Here's how the part is built. I have some questions about the finished solid (model axes, mm). Face numbers are marked on the shaded views. A direction names the side the tool comes from. Round coordinates to 2 decimals unless told otherwise and drop trailing zeros. Write each loop counter-clockwise with the first axis right and the second up, starting at its lowest first coordinate (ties: lowest second). Pieces come first, ordered by that corner, then holes. Notation, with made-up numbers: (85.25, -7.5) -> (127.25, -7.5) arc R14 ccw to (127.25, 19.5) -> close; hole circle Ø11 at (14.5, -2). An arc over 180 degrees is marked (long way). Answer in a Markdown table with one row per item.
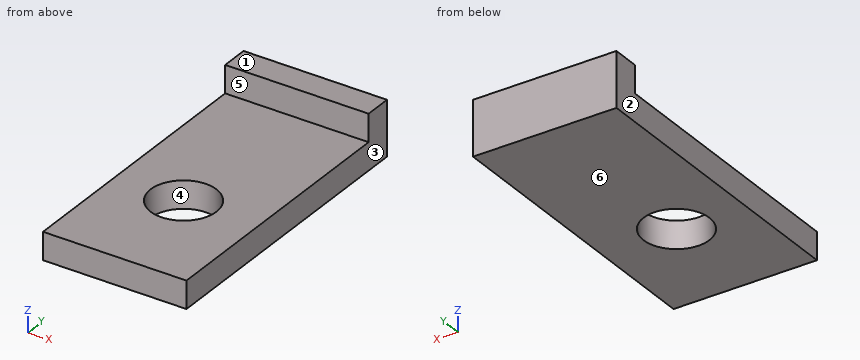
Autodesk Fusion 360 part; units mm, degrees
sketch "Esboço1" plane through (0, 0, 0) normal (0, 0, 1) x (1, 0, 0)
  line L0 (9, 9.5) -> (-9, 9.5)
  line L1 (-9, 9.5) -> (-9, -9.5)
  line L2 (-9, -9.5) -> (9, -9.5)
  line L3 (9, -9.5) -> (9, 9.5)
  line L4 (9, 9.5) -> (-9, -9.5) construction
  line L5 (-9, 9.5) -> (9, -9.5) construction
  line L6 (-7, -7.5) -> (7, -7.5)
  line L7 (7, -7.5) -> (7, 7.5)
  line L8 (7, 7.5) -> (-7, 7.5)
  line L9 (-7, 7.5) -> (-7, -7.5)
  dimension "d1" = 18
  dimension "d2" = 19
  dimension "d3" = -2
extrude "Extrusão1" add sketch "Esboço1" along normal blind 2 makes body 1
sketch "Esboço2" plane through (0, 0, 2) normal (0, 0, 1) x (-1, 0, 0)
  line L0 (7, 7.5) -> (7, -7.5)
  line L1 (7, -7.5) -> (-7, -7.5)
  line L2 (-7, -7.5) -> (-7, 7.5)
  line L3 (-7, 7.5) -> (7, 7.5)
  line L4 (-9, 9.5) -> (-9, -9.5)
  line L5 (-9, -9.5) -> (9, -9.5)
  line L6 (9, -9.5) -> (9, 9.5)
  line L7 (9, 9.5) -> (-9, 9.5)
  line L8 (-11, 9.5) -> (-11, -9.5)
  line L9 (-9, -11.5) -> (9, -11.5)
  line L10 (11, -9.5) -> (11, 9.5)
  line L11 (9, 11.5) -> (-9, 11.5)
  arc A0 (11, 9.5) -> (9, 11.5) centre (9, 9.5) ccw
  arc A1 (-9, 11.5) -> (-11, 9.5) centre (-9, 9.5) ccw
  arc A2 (-11, -9.5) -> (-9, -11.5) centre (-9, -9.5) ccw
  arc A3 (9, -11.5) -> (11, -9.5) centre (9, -9.5) ccw
  dimension "d7" = 2
extrude "Extrusão2" add sketch "Esboço2" along normal blind 2 contours L4 L5 L6 L7 | L8 L9 L10 L11 A0 A1 A2 A3 bodies 1
fillet "Arredondamento1" radius 2 4 edges at (-9, 9.5, 1) (-9, -9.5, 1) (9, 9.5, 1) (9, -9.5, 1) on bodies 1
fillet "Arredondamento2" radius 1 4 edges at (-7, 7.5, 2) (-7, -7.5, 2) (7, -7.5, 2) (7, 7.5, 2) on bodies 1
sketch "Esboço3" plane through (0, 0, 0) normal (0, 0, 1) x (1, 0, 0)
  circle A0 centre (-41, 0) radius 12
  line L0 (-57.5, -16.5) -> (-24.5, -16.5)
  line L1 (-24.5, -16.5) -> (-24.5, 16.5)
  line L2 (-24.5, 16.5) -> (-57.5, 16.5)
  line L3 (-57.5, 16.5) -> (-57.5, -16.5)
  line L4 (-57.5, -16.5) -> (-24.5, 16.5) construction
  line L5 (-24.5, -16.5) -> (-57.5, 16.5) construction
  point P0 (-41, 0)
  dimension "d14" = 24
  dimension "d15" = 33
  dimension "d16" = 33
extrude "Extrusão3" add sketch "Esboço3" along normal blind 1 separate body makes body 2
sketch "Esboço4" plane through (0, 0, 0) normal (0, 0, 1) x (1, 0, 0)
  line L0 (73, 0) -> (53, 0)
  line L1 (53, 0) -> (53, -20)
  line L2 (53, -20) -> (73, -20)
  line L3 (73, -20) -> (73, 0)
  line L4 (63, -20) -> (63, -12)
  circle A0 centre (63, -12) radius 2.4
  dimension "d19" = 20
  dimension "d20" = 20
  dimension "d21" = 8
  dimension "d22" = 4.8
extrude "Extrusão4" add sketch "Esboço4" along normal blind 10 separate body makes body 3
fillet "Arredondamento3" radius 6 2 edges at (73, -20, 5) (53, -20, 5) on bodies 3
sketch "Esboço5" plane through (0, 0, 10) normal (0, 0, 1) x (-1, 0, 0)
  circle A0 centre (-63, 12) radius 2.4
  arc A1 (-53, 14) -> (-59, 20) centre (-59, 14) ccw
  line L0 (-59, 20) -> (-67, 20)
  arc A2 (-67, 20) -> (-73, 14) centre (-67, 14) ccw
  line L1 (-73, 14) -> (-73, 0)
  line L2 (-73, 0) -> (-53, 0)
  line L3 (-53, 0) -> (-53, 14)
  line L4 (-53, 0) -> (-73, 0)
  line L5 (-73, 0) -> (-73, -2)
  line L6 (-73, -2) -> (-53, -2)
  line L7 (-53, -2) -> (-53, 0)
  dimension "d27" = 2
extrude "Extrusão5" add sketch "Esboço5" along normal blind 2 from surface at 1 separate body makes body 4
sketch "Esboço6" plane through (0, 0, 13) normal (0, 0, 1) x (-1, 0, 0)
  circle A0 centre (-63, 12) radius 2.4
  line L0 (-53, -2) -> (-53, 14)
  arc A1 (-53, 14) -> (-59, 20) centre (-59, 14) ccw
  line L1 (-59, 20) -> (-67, 20)
  arc A2 (-67, 20) -> (-73, 14) centre (-67, 14) ccw
  line L2 (-73, 14) -> (-73, -2)
  line L3 (-73, -2) -> (-53, -2)
  line L4 (-53, -2) -> (-73, -2)
  line L5 (-73, -2) -> (-73, 0)
  line L6 (-73, 0) -> (-53, 0)
  line L7 (-53, 0) -> (-53, -2)
extrude "Extrusão6" add sketch "Esboço6" along normal blind 2 contours L0 L2 L3 L4 L5 L6 L7 bodies 4
sketch "Esboço7" plane through (0, 0, 11) normal (0, 0, -1) x (1, 0, 0)
  circle A0 centre (63, 12) radius 2.4
  line L0 (53, 14) -> (53, -2)
  line L1 (53, -2) -> (73, -2)
  line L2 (73, -2) -> (73, 14)
  arc A1 (73, 14) -> (67, 20) centre (67, 14) ccw
  line L3 (67, 20) -> (59, 20)
  arc A2 (59, 20) -> (53, 14) centre (59, 14) ccw
  line L4 (58, -2) -> (68.4479, -2)
  line L5 (68.4479, -2) -> (68.4479, 19.8227)
  line L6 (68.4479, 19.8227) -> (58, 19.8227)
  line L7 (58, 19.8227) -> (58, -2)
extrude "Extrusão7" cut sketch "Esboço7" against normal blind 10 contours L0 L1 A1 L3 A2 L6 L7 | L1 L2 A1 L5 bodies 4
hidden bodies 1 2 3
1) I want a section at A-A, the plane x = 63. List the corners of the cut face in (y, z) for me.
Response:
| item | result |
|---|---|
| outline | (-19.82, 11) -> (-14.4, 11) -> (-14.4, 13) -> (-19.82, 13) -> close; (-9.6, 11) -> (2, 11) -> (2, 15) -> (0, 15) -> (0, 13) -> (-9.6, 13) -> close |
2) I need wall thicknesses on line 1 (Y direction, x = 63, z = 11.4); line 2 (X direction, y = -12, z = 12.3); line 3 (Z direction, x = 60.75, y = -17). Which ranges of each line are inside material? Lowest first, please. Write a range as [from, to].
Response:
| item | result |
|---|---|
| line 1 | y = [-19.82, -14.4], [-9.6, 2] |
| line 2 | x = [58, 60.6], [65.4, 68.45] |
| line 3 | z = [11, 13] |
3) We'd pull the mould along X, two halves only. Please class the marked faces 1, 2, 3 and 4: +X half, -X half, draft (parallel to the pull), parting line (faces both ways), or undercut.
Response:
| item | result |
|---|---|
| face 1 | draft |
| face 2 | -X half |
| face 3 | +X half |
| face 4 | undercut |
4) I want a section at B-B, the plane y = -12. List the corners of the cut face in (x, z) for me.
Response:
| item | result |
|---|---|
| outline | (58, 11) -> (60.6, 11) -> (60.6, 13) -> (58, 13) -> close; (65.4, 11) -> (68.45, 11) -> (68.45, 13) -> (65.4, 13) -> close |
5) Which directions (+Z, -Z, +X, -X, +Y, -Y) give clear straight access to the entire face, cutting with the end or side of a thin tool? Please do the marked faces 5 and 6.
Response:
| item | result |
|---|---|
| face 5 | +Z, +X, -X, -Y |
| face 6 | -Z, +X, -X, +Y, -Y |
6) I want a section at C-C, the plane z = 11.55. List the corners of the cut face in (x, y) for me, and give its area (3 significant figures).
Response:
| item | result |
|---|---|
| outline | (58, -19.82) -> (68.45, -19.82) -> (68.45, 2) -> (58, 2) -> close; hole circle Ø4.8 at (63, -12) |
| area | 210 mm^2 |
7) I want a section at D-D, the plane z = 14.75. List the corners of the cut face in (x, y) for me, and give its area (3 significant figures).
Response:
| item | result |
|---|---|
| outline | (58, 0) -> (68.45, 0) -> (68.45, 2) -> (58, 2) -> close |
| area | 20.9 mm^2 |
8) For pin 1 (6 mm diameter, centred on x = 63, y = -12, fed in from +Z); pin 2 (1.6 mm diameter, centred on x = 62.5, z = 14, fed in from -Y), each with a flat end and sliding along its axis, tell me the tip position at first contact or that it passes through.
Response:
| item | result |
|---|---|
| pin 1 | stops at z = 13 |
| pin 2 | stops at y = 0 |
